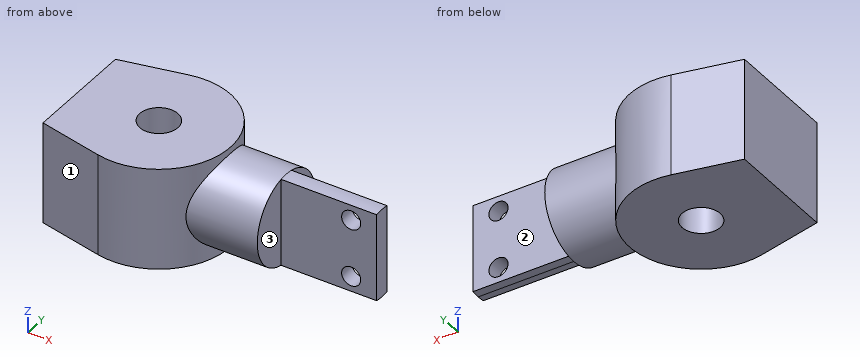
```python
from build123d import *

# Parameters (mm, degrees)
IZIM1_R                     = 6
Y_KSEKLIK_EKSTR_ZYON1_DEPTH = 16
Y_KSEKLIK_EKSTR_ZYON2_REACH = 67
IZIM2_R                     = 14
Y_KSEKLIK_EKSTR_ZYON3_DEPTH = 30
IZIM4_R                     = 3
KES_EKSTR_ZYON1_DEPTH       = 30


with BuildPart() as part:
    # Çizim1 → Yükseklik-Ekstrüzyon1 (new body, symmetric)
    with BuildSketch(Plane.XY):
        with BuildLine():
            Line((-25, 17.5), (-25, -17.5))
            Line((-25, -17.5), (-4.873971328, -21.965755245))
            ThreePointArc((-4.873971328, -21.965755245), (22.5, 0), (-4.873971328, 21.965755245))
            Line((-4.873971328, 21.965755245), (-25, 17.5))
        make_face()
        Circle(IZIM1_R, mode=Mode.SUBTRACT)
    extrude(amount=Y_KSEKLIK_EKSTR_ZYON1_DEPTH, both=True)

    # Çizim2 → Yükseklik-Ekstrüzyon2 (add, up to next)
    with BuildSketch(Plane(origin=(40, 0, 0), x_dir=(0, 0, -1), z_dir=(1, 0, 0)), mode=Mode.PRIVATE) as y_kseklik_ekstr_zyon2_sk1:
        Circle(IZIM2_R)
    y_kseklik_ekstr_zyon2_tool1 = extrude(y_kseklik_ekstr_zyon2_sk1.sketch, amount=-Y_KSEKLIK_EKSTR_ZYON2_REACH, mode=Mode.PRIVATE) - part.part
    add(y_kseklik_ekstr_zyon2_tool1.solids().sort_by_distance((40, 0, 0))[0])

    # Çizim3 → Yükseklik-Ekstrüzyon3 (add)
    with BuildSketch(Plane(origin=(40, 0, 0), x_dir=(0, 0, -1), z_dir=(1, 0, 0))):
        with BuildLine():
            ThreePointArc((-13.774977314, 2.5), (-14, 0), (-13.774977314, -2.5))
            Line((-13.774977314, -2.5), (13.774977314, -2.5))
            ThreePointArc((13.774977314, -2.5), (13.943630847, -1.255053307), (14, 0))
            ThreePointArc((14, 0), (13.943630847, 1.255053307), (13.774977314, 2.5))
            Line((13.774977314, 2.5), (-13.774977314, 2.5))
        make_face()
    extrude(amount=Y_KSEKLIK_EKSTR_ZYON3_DEPTH)

    # Çizim4 → Kes-Ekstrüzyon1 (cut)
    with BuildSketch(Plane(origin=(0, 2.5, 0), x_dir=(1, 0, 0), z_dir=(0, 1, 0))):
        with Locations((62, -9)):
            Circle(IZIM4_R)
        with Locations((62, 9)):
            Circle(IZIM4_R)
    extrude(amount=-KES_EKSTR_ZYON1_DEPTH, mode=Mode.SUBTRACT)


solid = part.part
```
The model under review builds one solid part; all positions refer to its coordinate system, in mm. Face numbers are marked on the shaded views. A direction names the side the tool comes from. Give positions to 0.01 mm unless a question says otherwise; leave off trailing zeros. Order: outer loops, then holes, each group sorted by start corner. A loop starts at its lowest first (then second) coordinate and runs counter-clockwise, first axis right, second up. Notation, with made-up numbers: (20.5, 23.5) - (45.5, 23.5) arc R22 cw to (45.5, 44.5) - close; hole circle Ø10 at (44, 32.25). An arc over 180 degrees is marked (long way). Use CSV: the item, a comma, the result in double quotes. Start each with the question number.
Q1. We need section D-D, the plane z = 0. Write out the cut boundary in (x, y).
Q2. We need section C-C, the plane x = 62. Write out the cut boundary in (y, z), and give its area (3 significant figures).
Q3. Tool access review of the marked faces 1, 2 and 3: name each direction out of +Z, -Z, +X, -X, +Y, -Y from which nothing blocks a thin tool from reaching the whole face with its end or side.
Q4. We need section B-B, the plane z = -9. Write out the cut boundary in (x, y), and give its area (3 significant figures).
Q5. To check wall thickness, follow line 1 along Z through (x, y) = (62, -0.7); line 2 along Y through (x, z) = (0, -4.5); line 3 along X through (y, z) = (-1, 9). State the ranges of each line that lie inside material, in increasing order. Write a range as [from, to].
Q6. Clearance check with flat-ended pins moving along their axes: pin 1 Ø14 at (x, z) = (60.5, 2.5) entering from -Y; pin 2 Ø3.5 at (y, z) = (-7, 5) entering from +X; pin 3 Ø1 at (x, y) = (33, -8) entering from +Z; pin 4 Ø5 at (x, z) = (62, 9) entering from -Y. State where each tip first meets the part, or that it passes through.
Q7. We need section A-A, the plane x = 0. Write out the cut boundary in (y, z).
Outcome:
1,outline,"(-25, -17.5) - (-4.87, -21.97) arc R22.5 ccw to (17.61, -14) - (40, -14) - (40, -2.5) - (70, -2.5) - (70, 2.5) - (40, 2.5) - (40, 14) - (17.61, 14) arc R22.5 ccw to (-4.87, 21.97) - (-25, 17.5) - close; hole circle Ø12 at (0, 0)"
2,outline,"(-2.5, -13.77) arc R14 ccw to (2.5, -13.77) - (2.5, -12) - (-2.5, -12) - close; (-2.5, -6) - (2.5, -6) - (2.5, 6) - (-2.5, 6) - close; (-2.5, 12) - (2.5, 12) - (2.5, 13.77) arc R14 ccw to (-2.5, 13.77) - close"
2,area,"79.3 mm^2"
3,face 1,"+Z, -Z, -X, -Y"
3,face 2,"+Z, -Z, +X, +Y"
3,face 3,"+Z, -Z, +X, -Y"
4,outline,"(-25, -17.5) - (-4.87, -21.97) arc R22.5 ccw to (19.78, -10.72) - (40, -10.72) - (40, -2.5) - (59, -2.5) - (59, 2.5) - (40, 2.5) - (40, 10.72) - (19.78, 10.72) arc R22.5 ccw to (-4.87, 21.97) - (-25, 17.5) - close; (65, -2.5) - (70, -2.5) - (70, 2.5) - (65, 2.5) - close; hole circle Ø12 at (0, 0)"
4,area,"2,210 mm^2"
5,line 1,"z = [-13.98, -12], [-6, 6], [12, 13.98]"
5,line 2,"y = [-22.5, -6], [6, 22.5]"
5,line 3,"x = [-25, -5.92], [5.92, 59], [65, 70]"
6,pin 1,"stops at y = -2.5"
6,pin 2,"stops at x = 40"
6,pin 3,"stops at z = 11.82"
6,pin 4,"passes through"
7,outline,"(-22.5, -16) - (-6, -16) - (-6, 16) - (-22.5, 16) - close; (6, -16) - (22.5, -16) - (22.5, 16) - (6, 16) - close"
